```python
from build123d import *

# Parameters (mm, degrees)
SKETCH1_R           = 6.9
SKETCH1_R_2         = 10.9
BOSS_EXTRUDE1_DEPTH = 7
BOSS_EXTRUDE2_DEPTH = 12
CUT_EXTRUDE1_DEPTH  = 13
BOSS_EXTRUDE3_DEPTH = 26
SKETCH5_R           = 7.973914392
SKETCH5_R_2         = 4
BOSS_EXTRUDE4_DEPTH = 1.5
BOSS_EXTRUDE5_START = -1.5
SKETCH6_R           = 8.491099949
SKETCH6_R_2         = 4
BOSS_EXTRUDE5_DEPTH = 1.5
SKETCH7_R           = 2.25
CUT_EXTRUDE2_DEPTH  = 99.438905233


with BuildPart() as part:
    # Sketch1 → Boss-Extrude1 (new body)
    with BuildSketch(Plane.XY):
        with BuildLine():
            ThreePointArc((-109.99286225, 64.498694041), (-120.238224228, 58.705152002), (-124.296770504, 47.657040238))
            Line((-124.296770504, 47.657040238), (-117.277493754, 25.812066819))
            ThreePointArc((-117.277493754, 25.812066819), (-114.348561566, 18.740999007), (-107.277493754, 15.812066819))
            add(Edge.make_bspline(
                [(-80.055270229, 25.812066819), (-90.16574855, 12.494826539), (-107.277493754, 15.812066819)],
                knots=[0, 0, 0, 1, 1, 1], degree=2))
            Line((-80.055270229, 25.812066819), (-80.055270229, 84.34418562))
            ThreePointArc((-80.055270229, 84.34418562), (-81.43033647, 86.24404293), (-83.664728026, 85.531470589))
            add(Edge.make_bspline(
                [(-109.99286225, 64.498694041), (-95.736844246, 69.471166394), (-91.130917767, 75.410465429), (-83.664728026, 85.531470589)],
                knots=[0, 0, 0, 0, 0.858728352, 0.858728352, 0.858728352, 0.858728352], degree=3))
        make_face()
        with Locations((-107.277493754, 25.812066819)):
            Circle(SKETCH1_R, mode=Mode.SUBTRACT)
        with Locations((-107.22999807, 47.657040238)):
            Circle(SKETCH1_R_2, mode=Mode.SUBTRACT)
    boss_extrude1 = extrude(amount=BOSS_EXTRUDE1_DEPTH)

    # Sketch2 → Boss-Extrude2 (add)
    with BuildSketch(Plane.XY.offset(7)):
        with BuildLine():
            Line((-85.055270217, 83.653678118), (-85.055270217, 20.583275514))
            add(Edge.make_bspline(
                [(-85.055270217, 20.583275514), (-82.371539661, 22.76114127), (-80.055270217, 25.812066834)],
                knots=[0, 0, 0, 1, 1, 1], degree=2))
            Line((-80.055270217, 25.812066834), (-80.055270229, 84.34418562))
            ThreePointArc((-80.055270229, 84.34418562), (-81.43033647, 86.24404293), (-83.664728026, 85.531470589))
            add(Edge.make_bspline(
                [(-83.664728026, 85.531470589), (-84.138702239, 84.888961408), (-84.601149423, 84.263304749), (-85.055270217, 83.653678118)],
                knots=[0, 0, 0, 0, 0.054514432, 0.054514432, 0.054514432, 0.054514432], degree=3))
        make_face()
    extrude(amount=BOSS_EXTRUDE2_DEPTH)

    # Mirror1: Boss-Extrude1 across plane
    add(boss_extrude1.mirror(Plane.XY.offset(13)))

    # Sketch3 → Cut-Extrude1 (cut)
    with BuildSketch(Plane(origin=(0, 0, 0), x_dir=(-1, 0, 0), z_dir=(0, 0, -1))):
        with BuildLine():
            Line((92.850529653, 74.397721592), (144.531216933, 88.865819457))
            Line((144.531216933, 88.865819457), (118.546118501, 29.760204905))
            add(Edge.make_bspline(
                [(107.22999807, 36.757040238), (116.864311021, 38.600442381), (118.546118501, 29.760204905)],
                knots=[0, 0, 0, 1, 1, 1], degree=2))
            ThreePointArc((107.22999807, 36.757040238), (99.522534155, 39.949576323), (96.32999807, 47.657040238))
            add(Edge.make_bspline(
                [(92.850529653, 74.397721592), (90.423550402, 60.160750292), (96.32999807, 47.657040238)],
                knots=[0, 0, 0, 1, 1, 1], degree=2))
        make_face()
    extrude(amount=-CUT_EXTRUDE1_DEPTH, mode=Mode.SUBTRACT)

    # Sketch4 → Boss-Extrude3 (add)
    with BuildSketch(Plane(origin=(0, 0, 0), x_dir=(-1, 0, 0), z_dir=(0, 0, -1))):
        with BuildLine():
            Line((83.132797407, 86.34418562), (85.055270217, 83.653678118))
            Line((85.055270217, 83.653678118), (85.055270214, 20.587782524))
            add(Edge.make_bspline(
                [(78.82999807, 27.533016311), (81.645897876, 23.355716893), (85.055270214, 20.587782524)],
                knots=[0, 0, 0, 1, 1, 1], degree=2))
            Line((78.82999807, 27.533016311), (78.82999807, 84.770259389))
            ThreePointArc((78.82999807, 84.770259389), (80.746261593, 86.200037671), (83.132797407, 86.34418562))
        make_face()
    extrude(amount=-BOSS_EXTRUDE3_DEPTH)

    # Sketch5 → Boss-Extrude4 (add)
    with BuildSketch(Plane.XY.offset(7)):
        with Locations((-107.277493754, 25.812066819)):
            Circle(SKETCH5_R)
        with Locations((-107.277493754, 25.812066819)):
            Circle(SKETCH5_R_2, mode=Mode.SUBTRACT)
    extrude(amount=-BOSS_EXTRUDE4_DEPTH)

    # Sketch6 → Boss-Extrude5 (add)
    with BuildSketch(Plane(origin=(0, 0, 19), x_dir=(-1, 0, 0), z_dir=(0, 0, -1)).offset(BOSS_EXTRUDE5_START)):
        with Locations((107.277493754, 25.812066819)):
            Circle(SKETCH6_R)
        with Locations(Location((107.277493754, 25.812066819, 0), (0, 0, 180))):
            Circle(SKETCH6_R_2, mode=Mode.SUBTRACT)
    extrude(amount=BOSS_EXTRUDE5_DEPTH)

    # Sketch7 → Cut-Extrude2 (cut, through all)
    with BuildSketch(Plane.ZY.offset(85.055270217)):
        with Locations(Location((13, 32.653678118, 0), (0, 0, 270))):
            Circle(SKETCH7_R)
        with Locations(Location((13, 52.653678118, 0), (0, 0, 270))):
            Circle(SKETCH7_R)
        with Locations(Location((13, 72.653678118, 0), (0, 0, 270))):
            Circle(SKETCH7_R)
    extrude(amount=-CUT_EXTRUDE2_DEPTH, mode=Mode.SUBTRACT)


solid = part.part
```
Work out the finished part from the listing and answer in its coordinate system (mm). A direction names the side the tool comes from. Coordinates: 2 decimals unless noted, no trailing zeros. Order: outer loops, then holes, each group sorted by start corner. A loop starts at its lowest first (then second) coordinate and runs counter-clockwise, first axis right, second up. Notation, with made-up numbers: (-11.5, -30) - (30.5, -30) arc R22 cw to (30.5, 5) - close; hole circle Ø9 at (62, 38.25). An arc over 180 degrees is marked (long way). Answer as a JSON object with one key per item and string values.
1. Find section B-B on z = 13. Count the separate pieces of the cut face and the enclosed holes in it, plus the area to 3 significant figures.
Output values:
{"separate pieces": "4", "enclosed holes": "0", "area": "302 mm²"}
2. The mould has two halves that part along Y. Classify faces 1 (the face through (-120.836, 36.887, 22.549)), 2 (the face through (-98, 41, 7)), 3 (the face through (-108.773, 19.076, 23.288)): +Y half, -Y half, draft (parallel to the pull), parting line (faces both ways), or undercut.
Output values:
{"face 1": "-Y half", "face 2": "draft", "face 3": "undercut"}
3. Consider line 1 (Z direction, x = -99, y = 22.5); line 2 (Y direction, x = -111, z = 24.25); line 3 (Y direction, x = -84, z = 12). Determine where each line is inside the solid, lowest interval first.
Output values:
{"line 1": "z = 0 to 7, 19 to 26", "line 2": "y = 16.53 to 20, 31.62 to 37.43, 57.88 to 64.3", "line 3": "y = 21.49 to 30.64, 34.67 to 50.64, 54.67 to 70.64, 74.67 to 85.13"}
4. Each of these flat-tipped pins is pushed along its axis until it touches: P1, Ø10, axis at x = -98, y = 60.5, coming from the -Z side; P2, Ø10.5, axis at x = -107.28, y = 25.81, coming from the +Z side; P3, Ø22, axis at x = -107.28, y = 25.81, coming from the -Z side; P4, Ø5, axis at y = 72.65, z = 13, coming from the -X side. Where does it stop, or does it pass through?
Output values:
{"P1": "stops at z = 19", "P2": "stops at z = 20.5", "P3": "stops at z = 0", "P4": "stops at x = -85.06"}
5. A tool of negligible diameter and unlimited length cuts with its end or side. For faces 4 (the face through (-110.2, 22.8, 20.5)), 5 (the face through (-96, 41, 19)), 6 (the face through (-108.773, 19.076, 2.712)), 7 (the face through (-118.12, 48.14, 22.55)), from which of +Z, -Z, +X, -X, +Y, -Y can it reach the whole face along a straight path? Write none if from no direction.
Output values:
{"face 4": "+Z", "face 5": "-X, +Y, -Y", "face 6": "-Z", "face 7": "+Z, -Z"}
6. Find section A-A on y = 42. Determine the outline of the cut face in (x, z), plus the area to 3 significant figures.
Output values:
{"outline": "(-122.48, 19) - (-116.55, 19) - (-116.55, 26) - (-122.48, 26) - close; (-97.91, 0) - (-78.83, 0) - (-78.83, 26) - (-97.91, 26) - (-97.91, 19) - (-85.06, 19) - (-85.06, 7) - (-97.91, 7) - close", "area": "383 mm²"}
